```python
from build123d import *

# Parameters (mm, degrees)
F0_W     = 750
F0_H     = 560
F1_DEPTH = 30
F4_DEPTH = 20
F5_DEPTH = 20
F6_W     = 560
F6_H     = 50
F7_DEPTH = 5


with BuildPart() as f1:
    # F0 (on Top) → F1 (new body)
    with BuildSketch(Plane.XY):
        Rectangle(F0_W, F0_H)
    extrude(amount=F1_DEPTH)

    # F3 (on face) → F4 (join)
    with BuildSketch(Plane(origin=(0, 280, 0), x_dir=(-1, 0, 0), z_dir=(0, 1, 0))):
        with BuildLine():
            Line((-188, 5), (375, 5))
            Line((375, 5), (375, 25))
            Line((375, 25), (-188, 25))
            ThreePointArc((-188, 25), (-198, 15), (-188, 5))
        make_face()
    extrude(amount=F4_DEPTH)

    # F2 (on face) → F5 (join)
    with BuildSketch(Plane.XZ.offset(280)):
        with BuildLine():
            Line((-375, 25), (-375, 5))
            Line((-375, 5), (188, 5))
            ThreePointArc((188, 5), (198, 15), (188, 25))
            Line((188, 25), (-375, 25))
        make_face()
    extrude(amount=F5_DEPTH)

    # F6 (on face) → F7 (join)
    with BuildSketch(Plane(origin=(-375, 0, 0), x_dir=(0, -1, 0), z_dir=(-1, 0, 0))):
        with Locations((0, 12.686171)):
            Rectangle(F6_W, F6_H)
    extrude(amount=F7_DEPTH)


solid = f1.part
```
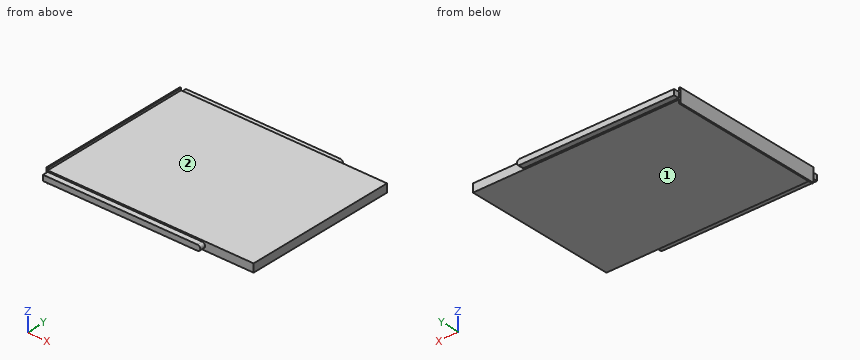
For this review, take the finished solid that the model builds, in its own axes (mm). Face numbers are marked on the shaded views. A direction names the side the tool comes from. Round coordinates to 2 decimals unless told otherwise and drop trailing zeros. Write each loop counter-clockwise with the first axis right and the second up, starting at its lowest first coordinate (ties: lowest second). Pieces come first, ordered by that corner, then holes. Notation, with made-up numbers: M 35,37.25 L 59,37.25 A28 cw 59,58.25 Z; hole C 45,31.25 d3. An arc over 180 degrees is marked long. One line per item, written item: value. Start each with the question number.
(1) Insertion check: pin 1 (3 mm diameter, centred on y = -184, z = -4.5, fed in from +X); pin 2 (10 mm diameter, centred on x = -43, y = -286.5, fed in from +Z); pin 3 (6 mm diameter, centred on x = 263.5, z = 17, fed in from -Y). Each pin has a flat end and moves straight along its axis. Give the tip position at first contact, or say it passes through.
(2) We need section B-B (x = -136). Give the boundary of the cut face in (y, z).
(3) We need section C-C (z = 15). Give the boundary of the cut face in (x, y), and give its area (3 significant figures).
(4) We need section A-A (y = 61.5). Give the boundary of the cut face in (x, z), and give its area (4 significant figures).
(5) We need section D-D (x = 244). Give the boundary of the cut face in (y, z).
(6) Machinability: for the marked faces 1 and 2, which of the approach directions +Z, -Z, +X, -X, +Y, -Y give a long, thin tool a straight path to every point of the face, cutting with its end or side? Answer none if there is none.
(7) Wall thickness on line 1 (Y direction, x = 337, z = 10.5); line 2 (Z direction, x = -160, y = -131); line 3 (X direction, y = 109, z = 35): over which ranges is each line inside the solid? List them lowest first.
Result:
1. pin 1: x = -375
1. pin 2: z = 25
1. pin 3: y = -280
2. outline: M -300,5 L -280,5 L -280,0 L 280,0 L 280,5 L 300,5 L 300,25 L 280,25 L 280,30 L -280,30 L -280,25 L -300,25 Z
3. outline: M -380,-280 L -375,-280 L -375,-300 L 198,-300 L 198,-280 L 375,-280 L 375,280 L 198,280 L 198,300 L -375,300 L -375,280 L -380,280 Z
3. area: 446,000 mm²
4. outline: M -380,-12.31 L -375,-12.31 L -375,0 L 375,0 L 375,30 L -375,30 L -375,37.69 L -380,37.69 Z
4. area: 22,750 mm²
5. outline: M -280,0 L 280,0 L 280,30 L -280,30 Z
6. face 1: -Z, +X, +Y, -Y
6. face 2: +Z, +X, +Y, -Y
7. line 1: -280 to 280
7. line 2: 0 to 30
7. line 3: -380 to -375
